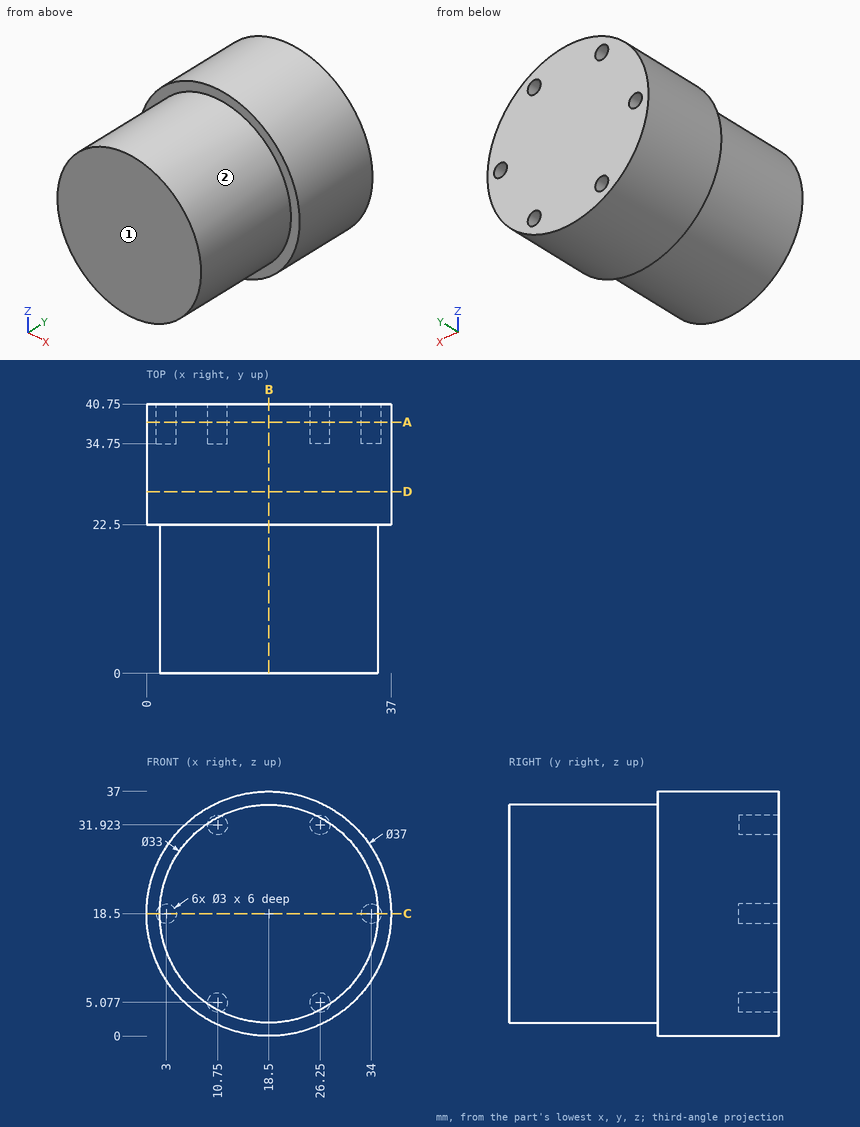
Design review of the part shown in the three views and the two pictorial views. Dimensions are in mm from the part's minimum x, y and z. A direction names the side the tool comes from. Round coordinates to 2 decimals unless told otherwise and drop trailing zeros. Loops run counter-clockwise (first coordinate to the right, second up) from the corner with the lowest first, then second, coordinate; pieces in that order, holes last. Notation, with made-up numbers: M 42,-32 L 83,-32 A8 cw 83,-28 Z; hole C 68,82 d6. An arc over 180 degrees is marked long. Answer as a JSON object with one key per item and string values.
Item 1: Wall thickness on L1, parallel to X at y = 38.85, z = 18.5; L2, parallel to Z at x = 10, y = 38 (1 decimal); L3, parallel to X at y = 33.5, z = 18: over which ranges is each line inside the solid? List them lowest first. Write a range as from..to.
Answer sheet:
{"L1": "x = 0..1.5, 4.5..32.5, 35.5..37", "L2": "z = 2.1..3.8, 6.4..30.6, 33.2..34.9", "L3": "x = 0.01..36.99"}
Item 2: We need section C-C on z = 18.5. Give the boundary of the cut face in (x, y), and give its area (3 significant figures).
Answer sheet:
{"outline": "M 0,22.5 L 2,22.5 L 2,0 L 35,0 L 35,22.5 L 37,22.5 L 37,40.75 L 35.5,40.75 L 35.5,34.75 L 32.5,34.75 L 32.5,40.75 L 4.5,40.75 L 4.5,34.75 L 1.5,34.75 L 1.5,40.75 L 0,40.75 Z", "area": "1,380 mm^2"}
Item 3: We need section D-D on y = 27.5. Give the boundary of the cut face in (x, z).
Answer sheet:
{"outline": "C 18.5,18.5 d37"}
Item 4: We need section A-A on y = 38. Give the boundary of the cut face in (x, z).
Answer sheet:
{"outline": "C 18.5,18.5 d37; hole C 3,18.5 d3; hole C 10.75,5.08 d3; hole C 10.75,31.92 d3; hole C 26.25,5.08 d3; hole C 26.25,31.92 d3; hole C 34,18.5 d3"}
Item 5: Clearance check with flat-ended pins moving along their axes: P1, Ø3.5, axis at x = 34, z = 18.5, coming from the +Y side; P2, Ø1.5, axis at x = 33.5, z = 18.5, coming from the +Y side; P3, Ø5, axis at y = 14, z = 7, coming from the +X side; P4, Ø10, axis at y = 5.5, z = 19, coming from the +X side. State where each tip first meets the part, or that it passes through.
Answer sheet:
{"P1": "stops at y = 40.75", "P2": "stops at y = 34.75", "P3": "stops at x = 32.33", "P4": "stops at x = 35"}
Item 6: Machinability: for the marked faces 1 and 2, which of the approach directions +Z, -Z, +X, -X, +Y, -Y give a long, thin tool a straight path to every point of the face, cutting with its end or side? Answer none if there is none.
Answer sheet:
{"face 1": "+Z, -Z, +X, -X, -Y", "face 2": "-Y"}
Item 7: We need section B-B on x = 18.5. Give the boundary of the cut face in (y, z).
Answer sheet:
{"outline": "M 0,2 L 22.5,2 L 22.5,0 L 40.75,0 L 40.75,37 L 22.5,37 L 22.5,35 L 0,35 Z"}
